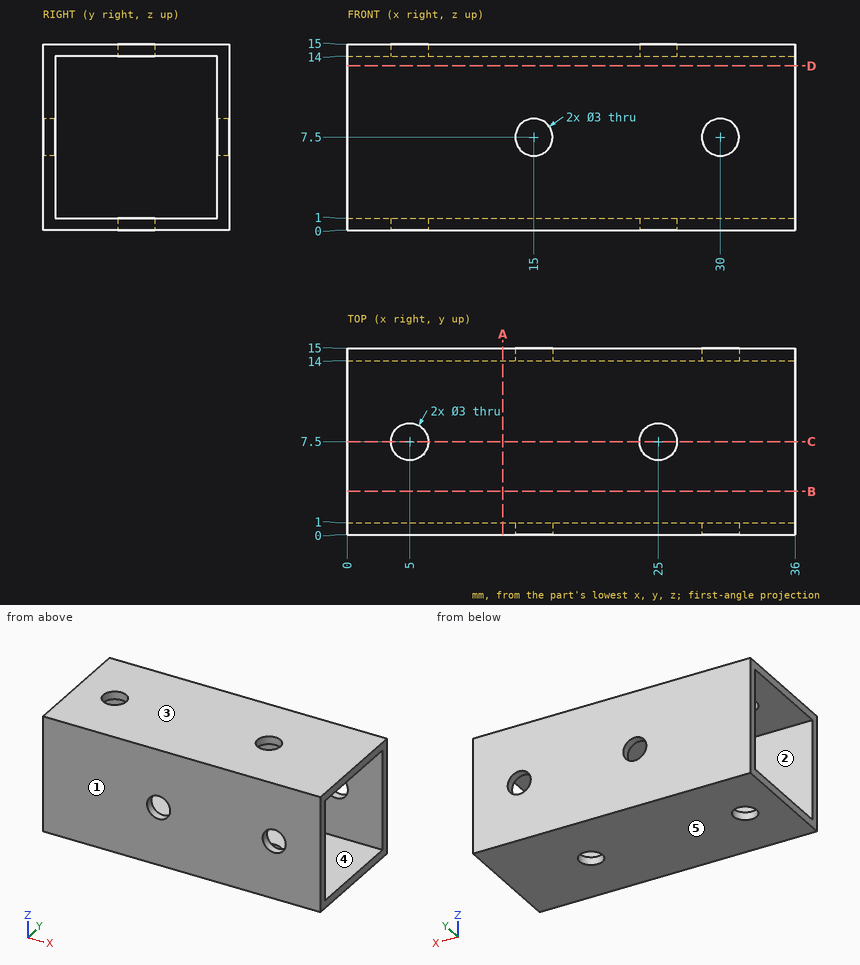
Job drawing, mm, ordinate dimensions from the low corner. One solid piece. A direction names the side the tool comes from. Give positions to 0.01 mm unless a question says otherwise; leave off trailing zeros. Order: outer loops, then holes, each group sorted by start corner. A loop starts at its lowest first (then second) coordinate and runs counter-clockwise, first axis right, second up. Notation, with made-up numbers: (43.5, 52.5) - (94.5, 52.5) arc R15 cw to (94.5, 71.5) - close; hole circle Ø11 at (80.25, 53.25). An arc over 180 degrees is marked (long way). Return JSON: item names as keys, results as strings.
1) Cut at B-B, the plane y = 3.5. Give the cut face in (x, z), plus the area to 3 significant figures.
Geometry says:
{"outline": "(0, 0) - (36, 0) - (36, 1) - (0, 1) - close; (0, 14) - (36, 14) - (36, 15) - (0, 15) - close", "area": "72.0 mm²"}
2) Cut at C-C, the plane y = 7.5. Give the cut face in (x, z), plus the area to 3 significant figures.
Geometry says:
{"outline": "(0, 0) - (3.5, 0) - (3.5, 1) - (0, 1) - close; (0, 14) - (3.5, 14) - (3.5, 15) - (0, 15) - close; (6.5, 0) - (23.5, 0) - (23.5, 1) - (6.5, 1) - close; (6.5, 14) - (23.5, 14) - (23.5, 15) - (6.5, 15) - close; (26.5, 0) - (36, 0) - (36, 1) - (26.5, 1) - close; (26.5, 14) - (36, 14) - (36, 15) - (26.5, 15) - close", "area": "60.0 mm²"}
3) Pull direction Z, two halves, no side cores. Call the marked faces 1, 2 and 3: pulls with the +Z half, pulls with the -Z half, needs draft (parallel to the pull), parting line crosses it, or undercut.
Geometry says:
{"face 1": "needs draft", "face 2": "undercut", "face 3": "pulls with the +Z half"}
4) Probe line 1 (X direction, y = 0.3, z = 7.5); line 2 (Z direction, x = 11, y = 12.75). List the from-to ranges inside material, lowest first. Write a range as from..to.
Geometry says:
{"line 1": "0..13.5, 16.5..28.5, 31.5..36", "line 2": "0..1, 14..15"}
5) Flat gauge pin, fed straight in: P1, Ø3.5, axis at x = 15, z = 7.5, coming from the +Y side. Where does the tip first touch, or does it go through?
Geometry says:
{"P1": "y = 15"}
6) 3-axis set-ups, long thin cutter, end or side, ignore diameter. For the marked faces 4 and 5: which of +Z, -Z, +X, -X, +Y, -Y reach the whole face in a straight line?
Geometry says:
{"face 4": "+X, -X", "face 5": "-Z, +X, -X, +Y, -Y"}
7) Cut at A-A, the plane x = 12.5. Give the cut face in (y, z).
Geometry says:
{"outline": "(0, 0) - (15, 0) - (15, 15) - (0, 15) - close; hole (1, 1) - (14, 1) - (14, 14) - (1, 14) - close"}
